CAD build for the part. Positions are in the model's coordinates, mm. Give positions to 0.01 mm unless a question says otherwise; leave off trailing zeros. Loops run counter-clockwise (first coordinate to the right, second up) from the corner with the lowest first, then second, coordinate; pieces in that order, holes last. Notation, with made-up numbers: (13, 86.5) - (67, 86.5) arc R21 ccw to (67, 94.5) - close; hole circle Ø4 at (79, 15). An arc over 180 degrees is marked (long way). Return JSON: item names as keys, results as strings.
from build123d import *

# Parameters (mm, degrees)
SKETCH1_W           = 418.07892
SKETCH1_H           = 415.925
BOSS_EXTRUDE1_DEPTH = 12.7
SKETCH2_W           = 418.07892
SKETCH2_H           = 79.68996
BOSS_EXTRUDE2_DEPTH = 12.7
SKETCH3_W           = 418.07892
SKETCH3_H           = 28.376126504
BOSS_EXTRUDE3_DEPTH = 12.7
BOSS_EXTRUDE4_DEPTH = 12.7
CHAMFER1_SIZE       = 304.8
CHAMFER1_SIZE_2     = 19.05
SKETCH5_W           = 12.7
SKETCH5_H           = 15.453987587
CUT_EXTRUDE1_DEPTH  = 5568.603780331


with BuildPart() as part:
    # Sketch1 → Boss-Extrude1 (new body)
    with BuildSketch(Plane.XY):
        with Locations((0, -5261.217030575)):
            Rectangle(SKETCH1_W, SKETCH1_H)
    extrude(amount=BOSS_EXTRUDE1_DEPTH)

    # Sketch2 → Boss-Extrude2 (add, through all)
    with BuildSketch(Plane(origin=(0, 0, 0), x_dir=(-1, 0, 0), z_dir=(0, 0, -1))):
        with Locations((0, -5509.024510575)):
            Rectangle(SKETCH2_W, SKETCH2_H)
    extrude(amount=-BOSS_EXTRUDE2_DEPTH)

    # Sketch3 → Boss-Extrude3 (add, through all)
    with BuildSketch(Plane(origin=(0, 0, 0), x_dir=(-1, 0, 0), z_dir=(0, 0, -1))):
        with Locations((0, -5039.066467323)):
            Rectangle(SKETCH3_W, SKETCH3_H)
    extrude(amount=-BOSS_EXTRUDE3_DEPTH)

    # Sketch4 → Boss-Extrude4 (add, through all)
    with BuildSketch(Plane(origin=(0, 0, 0), x_dir=(-1, 0, 0), z_dir=(0, 0, -1))):
        Polygon((209.038766336, -5447.352766987), (228.088766336, -5447.352766987), (228.088766336, -5548.869490575), (209.03946, -5548.869490575), align=None)
        Polygon((-209.03946, -5548.869490575), (-209.038766336, -5447.352766987), (-228.088766336, -5447.352766987), (-228.088766336, -5548.869490575), align=None)
    extrude(amount=-BOSS_EXTRUDE4_DEPTH)

    # Chamfer1
    # the kernel refuses this chamfer: 304.8, 19.05 mm, written as the material it adds along each edge
    with BuildSketch(Plane(origin=(-209.03946, -5447.352766987, 0), x_dir=(0.002399337658707147, 0.9999971215852571, 0), z_dir=(0, 0, 1))) as chamfer1_piece_1_section:
        Polygon((CHAMFER1_SIZE * 0.999997121585, CHAMFER1_SIZE * 0.00239933765871), (-CHAMFER1_SIZE_2 * 0.00239933765871, CHAMFER1_SIZE_2 * 0.999997121585), (0, 0), align=None)
    chamfer1_piece_1 = extrude(amount=12.7, mode=Mode.PRIVATE)
    chamfer1_piece_1 = split(chamfer1_piece_1, bisect_by=Plane(origin=(-228.088766336, -5325.682018196, 6.35), z_dir=(1, 0, 0)), keep=Keep.TOP, mode=Mode.PRIVATE)
    add(chamfer1_piece_1)
    with BuildSketch(Plane(origin=(209.03946, -5447.352766987, 0), x_dir=(0.8520963193143735, -0.5233850041899339, 0), z_dir=(0, 0, 1))) as chamfer1_piece_2_section:
        Polygon((CHAMFER1_SIZE_2 * 0.852096319314, CHAMFER1_SIZE_2 * 0.52338500419), (-CHAMFER1_SIZE * 0.52338500419, CHAMFER1_SIZE * 0.852096319314), (0, 0), align=None)
    chamfer1_piece_2 = extrude(amount=12.7, mode=Mode.PRIVATE)
    chamfer1_piece_2 = split(chamfer1_piece_2, bisect_by=Plane(origin=(228.088766336, -5325.682018196, 6.35), z_dir=(-1, 0, 0)), keep=Keep.TOP, mode=Mode.PRIVATE)
    add(chamfer1_piece_2)

    # Sketch5 → Cut-Extrude1 (cut, through all)
    with BuildSketch(Plane(origin=(228.088766336, 0, 0), x_dir=(0, 0, -1), z_dir=(1, 0, 0))):
        with Locations((-6.35, -5541.142496782)):
            Rectangle(SKETCH5_W, SKETCH5_H)
    extrude(amount=-CUT_EXTRUDE1_DEPTH, mode=Mode.SUBTRACT)


solid = part.part
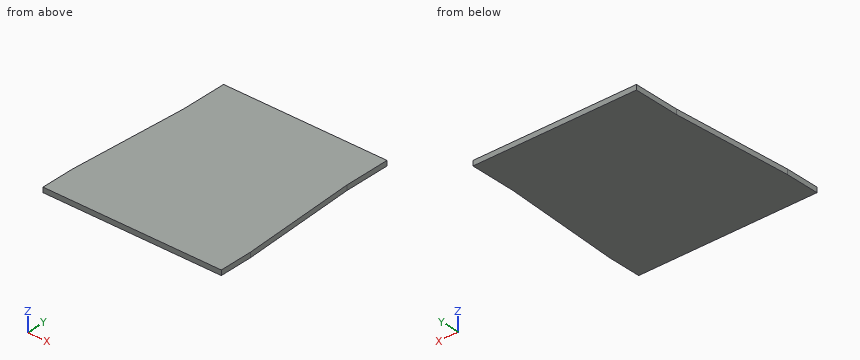
1. Cut at B-B, the plane y = -5099.5. Write the cut outline in (x, z), plus the area to 3 significant figures.
Values follow:
{"outline": "(-209.04, 0) - (209.04, 0) - (209.04, 12.7) - (-209.04, 12.7) - close", "area": "5,310 mm²"}
2. Drill centre lines: probe 1 along X at (y, z) = (-5098, 3); probe 2 along X at (y, z) = (-5213.5, 11.5). Where is each one in solid material? Low to high.
Values follow:
{"probe 1": "x = -209.04 to 209.04", "probe 2": "x = -213.47 to 213.47"}
3. Cut at C-C, the plane y = -5197.5. Write the cut outline in (x, z).
Values follow:
{"outline": "(-212.47, 0) - (212.47, 0) - (212.47, 12.7) - (-212.47, 12.7) - close"}
4. Cut at A-A, the plane z = 8. Write the cut outline in (x, y), plus the area to 3 significant figures.
Values follow:
{"outline": "(-228.09, -5533.42) - (228.09, -5533.42) - (228.09, -5447.34) - (209.04, -5142.55) - (209.04, -5024.88) - (-209.04, -5024.88) - (-209.04, -5142.55) - (-228.09, -5447.34) - close", "area": "222,000 mm²"}
5. Drop flat-ended pins along their axis: P1, Ø6.5, axis at y = -5107.5, z = 5.5, coming from the -X side; P2, Ø4, axis at y = -5089, z = 9, coming from the +X side; P3, Ø6, axis at y = -5161.5, z = 3.5, coming from the -X side. Give the stop position or say it passes through.
Values follow:
{"P1": "stops at x = -209.04", "P2": "stops at x = 209.04", "P3": "stops at x = -210.41"}
